```python
from build123d import *

# Parameters (mm, degrees)
F0_W     = 374.65
F0_H     = 337.693
F0_H_2   = 268.047813
F1_DEPTH = 254
F2_W     = 406.4
F2_H     = 1828.8
F3_DEPTH = 6.35


with BuildPart() as f1:
    # F0 (on Front) → F1 (new body)
    with BuildSketch(Plane.XZ):
        Polygon((-15.875, 0), (0, 0), (0, 1828.8), (-15.875, 1828.8), (-390.525, 1828.8), (-406.4, 1828.8), (-406.4, 0), (-390.525, 0), (-390.525, 114.730187), (-15.875, 114.730187), align=None)
        with Locations((-203.2, 299.451687)):
            Rectangle(F0_W, F0_H, mode=Mode.SUBTRACT)
        with Locations((-203.2, 653.019687)):
            Rectangle(F0_W, F0_H, mode=Mode.SUBTRACT)
        with Locations((-203.2, 1006.587687)):
            Rectangle(F0_W, F0_H, mode=Mode.SUBTRACT)
        with Locations((-203.2, 1360.155687)):
            Rectangle(F0_W, F0_H, mode=Mode.SUBTRACT)
        with Locations((-203.2, 1678.901093)):
            Rectangle(F0_W, F0_H_2, mode=Mode.SUBTRACT)
    extrude(amount=F1_DEPTH)

    # F2 (on face) → F3 (join)
    with BuildSketch(Plane(origin=(0, 0, 0), x_dir=(-1, 0, 0), z_dir=(0, 1, 0))):
        with Locations((203.2, 914.4)):
            Rectangle(F2_W, F2_H)
    extrude(amount=F3_DEPTH)


solid = f1.part
```
Build history of the part. All positions in model axes, mm. A direction names the side the tool comes from. Give positions to 0.01 mm unless a question says otherwise; leave off trailing zeros. Loops run counter-clockwise (first coordinate to the right, second up) from the corner with the lowest first, then second, coordinate; pieces in that order, holes last. Notation, with made-up numbers: (-7.5, 1) - (-0.5, 1) arc R23 ccw to (-0.5, 23) - close; hole circle Ø4 at (-1.75, 48). An arc over 180 degrees is marked (long way). Use a Markdown table: item, result.
(1) Band-saw the part on C-C (x = -97). Give the cut face in (y, z) (3 decimals), and give its area (3 significant figures).
Taken from the geometry:
| item | result |
|---|---|
| outline | (-254, 114.73) - (0, 114.73) - (0, 0) - (6.35, 0) - (6.35, 1828.8) - (-254, 1828.8) - (-254, 1812.925) - (0, 1812.925) - (0, 1544.877) - (-254, 1544.877) - (-254, 1529.002) - (0, 1529.002) - (0, 1191.309) - (-254, 1191.309) - (-254, 1175.434) - (0, 1175.434) - (0, 837.741) - (-254, 837.741) - (-254, 821.866) - (0, 821.866) - (0, 484.173) - (-254, 484.173) - (-254, 468.298) - (0, 468.298) - (0, 130.605) - (-254, 130.605) - close |
| area | 35,800 mm2 |
(2) Wall check: line 1 along Z through (x, y) = (-180, -241) (3 decimals); line 2 along X through (y, z) = (-238, 1221.5) (3 decimals); line 3 along Y through (x, z) = (-259.5, 1236). Give the ranges that are in metal, low to high.
Taken from the geometry:
| item | result |
|---|---|
| line 1 | 114.73 to 130.605, 468.298 to 484.173, 821.866 to 837.741, 1175.434 to 1191.309, 1529.002 to 1544.877, 1812.925 to 1828.8 |
| line 2 | -406.4 to -390.525, -15.875 to 0 |
| line 3 | 0 to 6.35 |
(3) Drop flat-ended pins along their axis: pin 1 Ø4 at (x, y) = (-312, -106) entering from -Z; pin 2 Ø2 at (y, z) = (-146, 1187.5) entering from +X; pin 3 Ø1 at (x, z) = (-141, 611.5) entering from -Y. Give the stop position or say it passes through.
Taken from the geometry:
| item | result |
|---|---|
| pin 1 | z = 114.73 |
| pin 2 | x = 0 |
| pin 3 | y = 0 |
(4) Which spindle directions (+Z, -Z, +X, -X, +Y, -Y) get a long thin tool onto all of the face, cutting with end or side? Do faces 1 (the face through (-201, 0, 58)), 2 (the face through (-206, -125, 1812.925)). Say none if no direction does.
Taken from the geometry:
| item | result |
|---|---|
| face 1 | -Z, -Y |
| face 2 | -Y |
(5) Band-saw the part on B-B (z = 871). Give the cut face in (x, y) (3 decimals), and give its area (3 significant figures).
Taken from the geometry:
| item | result |
|---|---|
| outline | (-406.4, -254) - (-390.525, -254) - (-390.525, 0) - (-15.875, 0) - (-15.875, -254) - (0, -254) - (0, 6.35) - (-406.4, 6.35) - close |
| area | 10,600 mm2 |
(6) Pull direction X, two halves, no side cores. Call faces 3 (the face through (-201, 0, 655)), 4 (the face through (0, -126, 902)), 5 (the face through (-202, 1, 0)), 6 (the face through (-206, -125, 114.73)): +X half, -X half, draft (parallel to the pull), parting line (faces both ways), or undercut.
Taken from the geometry:
| item | result |
|---|---|
| face 3 | undercut |
| face 4 | +X half |
| face 5 | draft |
| face 6 | undercut |
(7) Band-saw the part on A-A (y = -22.5). Give the cut face in (x, z) (3 decimals), and give its area (4 significant figures).
Taken from the geometry:
| item | result |
|---|---|
| outline | (-406.4, 0) - (-390.525, 0) - (-390.525, 114.73) - (-15.875, 114.73) - (-15.875, 0) - (0, 0) - (0, 1828.8) - (-406.4, 1828.8) - close; hole (-390.525, 130.605) - (-15.875, 130.605) - (-15.875, 468.298) - (-390.525, 468.298) - close; hole (-390.525, 484.173) - (-15.875, 484.173) - (-15.875, 821.866) - (-390.525, 821.866) - close; hole (-390.525, 837.741) - (-15.875, 837.741) - (-15.875, 1175.434) - (-390.525, 1175.434) - close; hole (-390.525, 1191.309) - (-15.875, 1191.309) - (-15.875, 1529.002) - (-390.525, 1529.002) - close; hole (-390.525, 1544.877) - (-15.875, 1544.877) - (-15.875, 1812.925) - (-390.525, 1812.925) - close |
| area | 93,750 mm2 |
